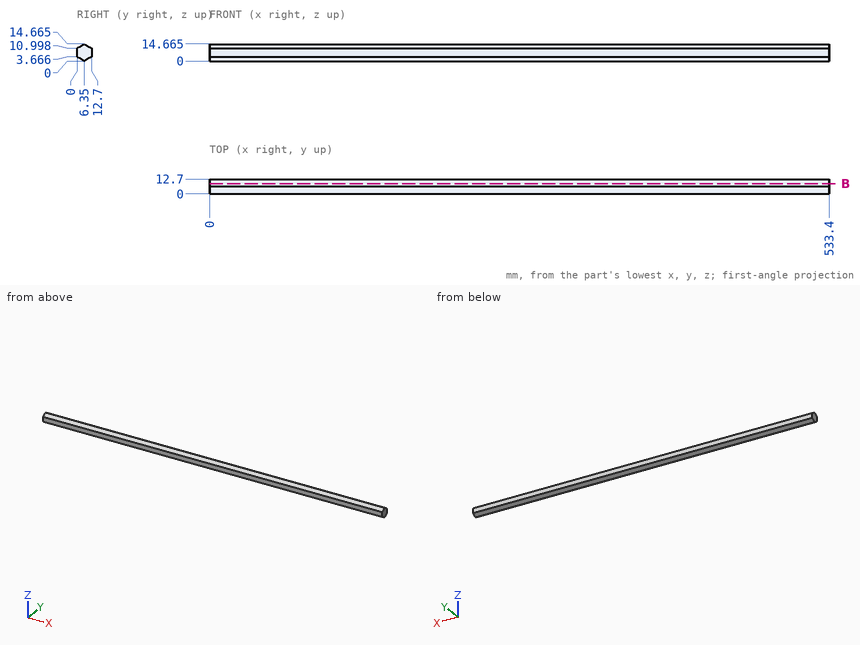
For this review, use the dimensioned drawing (mm, ordinates from the lowest corner) and the shaded views. Coordinates: 2 decimals unless noted, no trailing zeros. Order: outer loops, then holes, each group sorted by start corner. A loop starts at its lowest first (then second) coordinate and runs counter-clockwise, first axis right, second up. Notation, with made-up numbers: (-29.75, 13) - (4.25, 13) arc R21 cw to (4.25, 37) - close; hole circle Ø10 at (24, 0.5). An arc over 180 degrees is marked (long way). Answer as a JSON object with one key per item and string values. Group by question number.
1. For probe 1 along Z at (x, y) = (245, 11.5) (1 decimal); probe 2 along Y at (x, z) = (315, 13.5) (1 decimal); probe 3 along Y at (x, z) = (467.5, 2) (1 decimal), list the stretches that pass through material, from the lowest coordinate up.
2. Clearance check with flat-ended pins moving along their axes: P1, Ø5, axis at y = 9, z = 9, coming from the -X side; P2, Ø1, axis at x = 462.5, z = 12.5, coming from the +Y side (1 decimal); P3, Ø1.5, axis at x = 376.5, y = 2.5, coming from the +Z side (1 decimal). State where each tip first meets the part, or that it passes through.
3. We need section B-B on y = 8.75. State the section outline as (x, z) points (1 decimal).
Final values:
{
 "1": {"probe 1": "3 to 11.7", "probe 2": "4.3 to 8.4", "probe 3": "2.9 to 9.8"},
 "2": {"P1": "x = 0", "P2": "y = 11", "P3": "z = 12.9"},
 "3": {"outline": "(0, 1.4) - (533.4, 1.4) - (533.4, 13.3) - (0, 13.3) - close"}
}
